CAD build for the part. Positions are in the model's coordinates, mm. Face numbers are marked on the shaded views. A direction names the side the tool comes from. Give positions to 0.01 mm unless a question says otherwise; leave off trailing zeros. Loops run counter-clockwise (first coordinate to the right, second up) from the corner with the lowest first, then second, coordinate; pieces in that order, holes last. Notation, with made-up numbers: M 0.5,39.5 L 51.5,39.5 A19 ccw 51.5,65.5 Z; hole C 61.25,85 d4. An arc over 180 degrees is marked long. One line per question, with ' | ' between items.
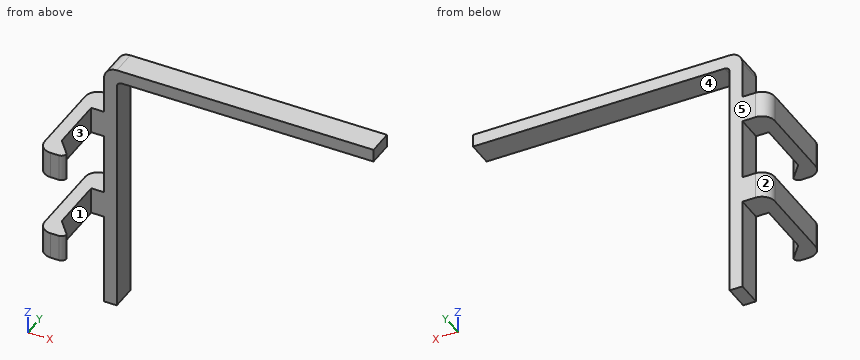
```python
from build123d import *

# Parameters (mm, degrees)
F1_DEPTH = 10
F2_W     = 5
F2_H     = 10.4262067128
F3_DEPTH = 30
F4_R     = 4.99999
F6_DEPTH = 10.4262067128
F8_DEPTH = 10.4262067128


# Not quite as in the source:
# - a fillet or chamfer is up to 0.001 mm smaller than in the source, because OpenCascade refuses the exact size


with BuildPart() as f1:
    # F0 (on Front) → F1 (new body)
    with BuildSketch(Plane.XZ):
        with BuildLine():
            Line((-5, -51.3071772588), (0, -51.3071772588))
            Line((0, -51.3071772588), (0, 42.0990820395))
            ThreePointArc((0, 42.0990820395), (0.5857864376, 43.5132956019), (2, 44.0990820395))
            Line((2, 44.0990820395), (100.4062592983, 44.0990820395))
            Line((100.4062592983, 44.0990820395), (100.4062592983, 49.0990820395))
            Line((100.4062592983, 49.0990820395), (0, 49.0990820395))
            ThreePointArc((0, 49.0990820395), (-3.5355339059, 47.6346159455), (-5, 44.0990820395))
            Line((-5, 44.0990820395), (-5, 29.6768955886))
            Line((-5, 29.6768955886), (-15, 29.6768955886))
            Line((-15, 29.6768955886), (-15, 19.2506888759))
            Line((-15, 19.2506888759), (-5, 19.2506888759))
            Line((-5, 19.2506888759), (-5, -4.6830929693))
            Line((-5, -4.6830929693), (-15, -4.6830929693))
            Line((-15, -4.6830929693), (-15, -15.1092996821))
            Line((-15, -15.1092996821), (-5, -15.1092996821))
            Line((-5, -15.1092996821), (-5, -51.3071772588))
        make_face()
    extrude(amount=F1_DEPTH)

    # F2 (on face) → F3 (join)
    with BuildSketch(Plane.XZ.offset(10)):
        with Locations((-12.5, 24.4637922322)):
            Rectangle(F2_W, F2_H)
        with Locations((-12.5, -9.8961963257)):
            Rectangle(F2_W, F2_H)
    extrude(amount=F3_DEPTH)

    # F4 (radius 5 in the source; OpenCascade refuses exactly that, so slightly less here)
    f4_edges = [f1.edges().sort_by_distance(p)[0] for p in [
        (-15, -40, 24.463792),
        (-15, -40, -9.896196),
        (-15, 0, 24.463792),
        (-15, 0, -9.896196),
    ]]
    fillet(f4_edges, radius=F4_R)

    # F5 (on face) → F6 (join, through all)
    with BuildSketch(Plane(origin=(0, 0, -15.1092996821), x_dir=(1, 0, 0), z_dir=(0, 0, -1))):
        with BuildLine():
            Line((-6.8065949231, 40), (-10, 40))
            Line((-10, 40), (-10, 31.8107408419))
            Line((-10, 31.8107408419), (-4.8065949231, 38))
            ThreePointArc((-4.8065949231, 38), (-5.3923813608, 39.4142135624), (-6.8065949231, 40))
        make_face()
    extrude(amount=-F6_DEPTH)

    # F7 (on face) → F8 (join, through all)
    with BuildSketch(Plane(origin=(0, 0, 19.2506888759), x_dir=(1, 0, 0), z_dir=(0, 0, -1))):
        with BuildLine():
            Line((-6.8065949231, 40), (-10, 40))
            Line((-10, 40), (-10, 31.8107408419))
            Line((-10, 31.8107408419), (-4.8065949231, 38))
            ThreePointArc((-4.8065949231, 38), (-5.3923813608, 39.4142135624), (-6.8065949231, 40))
        make_face()
    extrude(amount=-F8_DEPTH)


solid = f1.part
```
Item 1: Mould opens along Y. For the marked faces 3, 4 and 5 say: pulls with the +Y half, pulls with the -Y half, needs draft (parallel to the pull), parting line crosses it, or undercut.
Conclusion:
face 3: undercut | face 4: needs draft | face 5: pulls with the +Y half
Item 2: 3-axis set-ups, long thin cutter, end or side, ignore diameter. For the marked faces 1 and 2: which of +Z, -Z, +X, -X, +Y, -Y reach the whole face in a straight line?
Conclusion:
face 1: +Z, -Z, +X | face 2: +Z, -Z, -X, +Y
Item 3: Saw through at A-A on y = -28. Give the cut face in (x, z).
Conclusion:
outline: M -15,-15.11 L -10,-15.11 L -10,-4.68 L -15,-4.68 Z; M -15,19.25 L -10,19.25 L -10,29.68 L -15,29.68 Z
Item 4: Saw through at B-B on y = -7. Give the cut face in (x, z), and give its area (3 significant figures).
Conclusion:
outline: M -15,-15.11 L -5,-15.11 L -5,-51.31 L 0,-51.31 L 0,42.1 A2 cw 2,44.1 L 100.41,44.1 L 100.41,49.1 L 0,49.1 A5 ccw -5,44.1 L -5,29.68 L -15,29.68 L -15,19.25 L -5,19.25 L -5,-4.68 L -15,-4.68 Z | area: 1,210 mm²
Item 5: Saw through at C-C on z = -10. Give the cut face in (x, y).
Conclusion:
outline: M -15,-35 A5 ccw -10,-40 L -6.81,-40 A2 ccw -4.81,-38 L -10,-31.81 L -10,-10 L 0,-10 L 0,0 L -10,0 A5 ccw -15,-5 Z
Item 6: Drill centre lines: line 1 along Z through (x, y) = (87, -5); line 2 along Y through (x, z) = (2, 45); line 3 along X through (y, z) = (-8, -7). Where is each one in solid material? Low to high. Write a range as [from, to].
Conclusion:
line 1: [44.1, 49.1] | line 2: [-10, 0] | line 3: [-15, 0]
Item 7: Drop flat-ended pins along their axis: P1, Ø3, axis at y = -25.5, z = -7.5, coming from the +X side; P2, Ø6, axis at y = -10, z = -31, coming from the -X side; P3, Ø11, axis at x = 60, y = -3, coming from the -Z side. Give the stop position or say it passes through.
Conclusion:
P1: x = -10 | P2: x = -5 | P3: z = 44.1
Item 8: Saw through at D-D on x = 78.5. Give the cut face in (y, z).
Conclusion:
outline: M -10,44.1 L 0,44.1 L 0,49.1 L -10,49.1 Z
